For this review, take the finished solid that the model builds, in its own axes (mm). Give positions to 0.01 mm unless a question says otherwise; leave off trailing zeros. Loops run counter-clockwise (first coordinate to the right, second up) from the corner with the lowest first, then second, coordinate; pieces in that order, holes last. Notation, with made-up numbers: (50.25, -10.5) -> (95.25, -10.5) arc R31 ccw to (95.25, 16.5) -> close; hole circle Ø5 at (63.5, -26.75). An arc over 180 degrees is marked (long way). One line per question, with ' | ' between items. Start each with the question number.
(1) Consider section A-A (y = 17.5). Write out the cut boundary in (x, z).
(2) Insertion check: P1, Ø5.5, axis at x = -13, z = 4.5, coming from the +Y side; P2, Ø0.5, axis at x = 1, y = 4.5, coming from the +Z side; P3, Ø12, axis at x = -0.5, y = 43.5, coming from the +Z side; P4, Ø1, axis at x = -7, y = 24, coming from the +Z side (3 decimals). Each pin has a flat end and moves straight along its axis. Give the tip position at first contact, or say it passes through.
(3) Consider section B-B (x = 16.5). Write out the cut boundary in (y, z).
(4) Consider section D-D (x = -8.5). Write out the cut boundary in (y, z).
(5) Consider section C-C (z = -9.2). Write out the cut boundary in (x, y), and give its area (3 significant figures).
(6) Wall thickness on probe 1 along X at (y, z) = (52.5, -0.5); probe 2 along Y at (x, z) = (12.5, -7); probe 3 along X at (y, z) = (1, 18): over which ranges is each line inside the solid? List them lowest first.
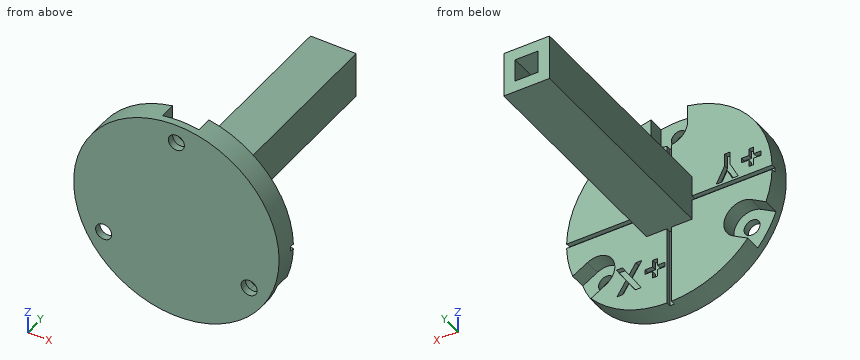
from build123d import *

# Parameters (mm, degrees)
SKETCH1_R                     = 22.5
PLATE_DEPTH                   = 5
OPENING_START                 = 1.5
OPENING_FOR_SCREW_DEPTH       = 5
SKETCH7_R                     = 1.75
SCREW_HOLE_DEPTH              = 5
CIRPATTERN20_COUNT            = 3
SKETCH10_W                    = 45
SKETCH10_H                    = 1
SKETCH10_W_2                  = 1
SKETCH10_H_2                  = 45
CUT_EXTRUDE5_DEPTH            = 1
CUT_EXTRUDE6_DEPTH            = 1
SKETCH12_W                    = 10
SKETCH12_H                    = 10
SKETCH12_W_2                  = 5
SKETCH12_H_2                  = 5
TOOL_CONNECT_PIECE_DEPTH      = 50
TOOL_CONNECT_PIECE_DEPTH_BACK = 1


with BuildPart() as part:
    # Sketch1 → plate (new body)
    with BuildSketch(Plane(origin=(0, 0, 0), x_dir=(1, 0, 0), z_dir=(0, 1, 0))):
        Circle(SKETCH1_R)
    extrude(amount=PLATE_DEPTH)

    # Sketch6 → opening for screw (cut)
    with BuildSketch(Plane(origin=(0, 5, 0), x_dir=(1, 0, 0), z_dir=(0, 1, 0)).offset(OPENING_START)):
        with BuildLine():
            Line((-4, -22.5), (-4, -18.4))
            ThreePointArc((-4, -18.4), (0, -14.4), (4, -18.4))
            Line((4, -18.4), (4, -22.5))
            ThreePointArc((4, -22.5), (0, -26.5), (-4, -22.5))
        make_face()
    opening_for_screw = extrude(amount=-OPENING_FOR_SCREW_DEPTH, mode=Mode.SUBTRACT)

    # Sketch7 → screw hole (cut)
    with BuildSketch(Plane(origin=(0, 1.5, 0), x_dir=(1, 0, 0), z_dir=(0, 1, 0))):
        with Locations((0, -18.4)):
            Circle(SKETCH7_R)
    screw_hole = extrude(amount=-SCREW_HOLE_DEPTH, mode=Mode.SUBTRACT)

    # CirPattern20: opening for screw, screw hole ×3 about axis
    cirpattern20_axis = Axis((0, 0, 0), (0, 1, 0))
    for i in range(1, CIRPATTERN20_COUNT):
        add(opening_for_screw.rotate(cirpattern20_axis, i * 360 / CIRPATTERN20_COUNT), mode=Mode.SUBTRACT)
        add(screw_hole.rotate(cirpattern20_axis, i * 360 / CIRPATTERN20_COUNT), mode=Mode.SUBTRACT)

    # Sketch10 → Cut-Extrude5 (cut)
    with BuildSketch(Plane(origin=(0, 5, 0), x_dir=(1, 0, 0), z_dir=(0, 1, 0))):
        Rectangle(SKETCH10_W, SKETCH10_H)
        Rectangle(SKETCH10_W_2, SKETCH10_H_2)
    extrude(amount=-CUT_EXTRUDE5_DEPTH, mode=Mode.SUBTRACT)

    # Sketch11 → Cut-Extrude6 (cut)
    with BuildSketch(Plane(origin=(0, 5, 0), x_dir=(1, 0, 0), z_dir=(0, 1, 0))):
        Polygon((2.616666667, 13.742425761), (2.616666667, 15.289220632), (3.675, 15.289220632), (3.675, 13.742425761), (5.303205128, 13.742425761), (5.303205128, 12.684092427), (3.675, 12.684092427), (3.675, 11.137297556), (2.616666667, 11.137297556), (2.616666667, 12.684092427), (0.988461538, 12.684092427), (0.988461538, 13.742425761), align=None)
        Polygon((6.136388221, 16.510374479), (7.479657452, 16.510374479), (8.806390224, 14.471301963), (10.135667067, 16.510374479), (11.480208333, 16.510374479), (9.47802484, 13.43968137), (11.6125, 10.160374479), (10.269230769, 10.160374479), (8.806390224, 12.409332812), (7.339733574, 10.160374479), (5.995192308, 10.160374479), (8.134755609, 13.440953405), align=None)
        Polygon((-18.458103671, -3.794817635), (-18.458103671, -2.248022763), (-17.399770338, -2.248022763), (-17.399770338, -3.794817635), (-15.771565209, -3.794817635), (-15.771565209, -4.853150968), (-17.399770338, -4.853150968), (-17.399770338, -6.39994584), (-18.458103671, -6.39994584), (-18.458103671, -4.853150968), (-20.086308799, -4.853150968), (-20.086308799, -3.794817635), align=None)
        Polygon((-15.07957803, -1.026868917), (-13.811358879, -1.026868917), (-12.677975466, -3.254202651), (-11.544592052, -1.026868917), (-10.276372902, -1.026868917), (-12.108103671, -4.626728693), (-12.108103671, -7.376868917), (-13.247847261, -7.376868917), (-13.247847261, -4.626728693), align=None)
    extrude(amount=-CUT_EXTRUDE6_DEPTH, mode=Mode.SUBTRACT)

    # Sketch12 → tool connect piece (add, two sides)
    with BuildSketch(Plane(origin=(0, 5, 0), x_dir=(1, 0, 0), z_dir=(0, 1, 0))) as tool_connect_piece_sk:
        Rectangle(SKETCH12_W, SKETCH12_H)
        Rectangle(SKETCH12_W_2, SKETCH12_H_2, mode=Mode.SUBTRACT)
    extrude(amount=TOOL_CONNECT_PIECE_DEPTH)
    extrude(tool_connect_piece_sk.sketch, amount=-TOOL_CONNECT_PIECE_DEPTH_BACK)


solid = part.part
A:
1) outline: (-5, -5) -> (5, -5) -> (5, 5) -> (-5, 5) -> close; hole (-2.5, -2.5) -> (2.5, -2.5) -> (2.5, 2.5) -> (-2.5, 2.5) -> close
2) P1: stops at y = 5 | P2: stops at z = 14.6 | P3: stops at z = 5 | P4: passes through
3) outline: (0, -15.3) -> (5, -15.3) -> (5, -14.15) -> (1.5, -14.15) -> (1.5, -10.86) -> (0, -10.86) -> close; (0, -7.54) -> (1.5, -7.54) -> (1.5, -5.24) -> (5, -5.24) -> (5, -0.5) -> (4, -0.5) -> (4, 0.5) -> (5, 0.5) -> (5, 15.3) -> (0, 15.3) -> close
4) outline: (0, -20.83) -> (5, -20.83) -> (5, -0.5) -> (4, -0.5) -> (4, 0.5) -> (5, 0.5) -> (5, 20.83) -> (0, 20.83) -> close
5) outline: (-20.53, 0) -> (-17.68, 0) -> (-17.68, 1.5) -> (-20.53, 1.5) -> close; (-14.18, 0) -> (14.18, 0) -> (14.18, 1.5) -> (11.93, 1.5) -> (11.93, 5) -> (0.5, 5) -> (0.5, 4) -> (-0.5, 4) -> (-0.5, 5) -> (-11.93, 5) -> (-11.93, 1.5) -> (-14.18, 1.5) -> close; (17.68, 0) -> (20.53, 0) -> (20.53, 1.5) -> (17.68, 1.5) -> close | area: 134 mm^2
6) probe 1: x = -5 to -2.5, 2.5 to 5 | probe 2: y = 0 to 5 | probe 3: x = -13.5 to -1.7, 1.7 to 13.5
